Verification items for this drawing (mm, ordinates from the low corner). Round coordinates to 2 decimals unless told otherwise and drop trailing zeros. Loops run counter-clockwise (first coordinate to the right, second up) from the corner with the lowest first, then second, coordinate; pieces in that order, holes last. Notation, with made-up numbers: (69.5, -32) - (103.5, -32) arc R21 ccw to (103.5, -9) - close; hole circle Ø3 at (-33.75, 74). An arc over 180 degrees is marked (long way). Answer in a Markdown table with one row per item. Add a question column.
(1) Mould release check, pull along X, two halves, no side actions. Record for the marked faces 1, 2 and 3: +X half, -X half, draft (parallel to the pull), parting line (faces both ways), or undercut.
(2) Cross-section at D-D on z = 8.5. Enter the section's corners in (x, y), then the cut area to 3 significant figures.
(3) Cross-section at A-A on z = 3. Enter the section's corners in (x, y).
(4) Thickness scan on line 1 along Y through (x, z) = (6, 12); line 2 along Z through (x, y) = (5, 7.25); line 3 along Z through (x, y) = (6.25, 5.75). Record the ranges inside material, lowest first.
(5) Gauge pin test, flat ends, axial feed: pin 1 (2.5 mm diameter, centred on x = 6, y = 6, fed in from +Z); pin 2 (1.5 mm diameter, centred on y = 2.5, z = 8, fed in from +X); pin 3 (3 mm diameter, centred on x = 8, y = 2.5, fed in from -Z). Record the tip position at first contact, or that the pin passes through.
(6) Cross-section at C-C on y = 6. Enter the section's corners in (x, z).
(7) Cross-section at B-B on x = 6. Enter the section's corners in (y, z).
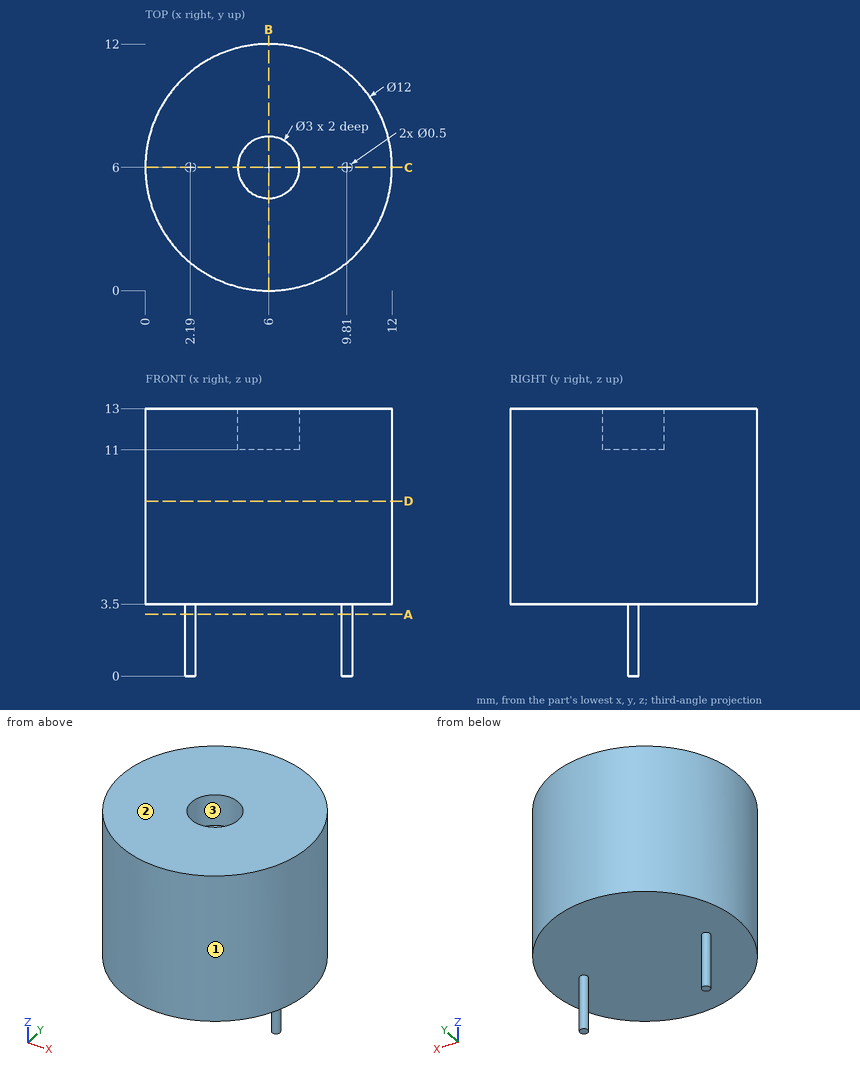
Answers:
| question | item | result |
|---|---|---|
| 1 | face 1 | parting line |
| 1 | face 2 | draft |
| 1 | face 3 | undercut |
| 2 | outline | circle Ø12 at (6, 6) |
| 2 | area | 113 mm^2 |
| 3 | outline | circle Ø0.5 at (2.19, 6); circle Ø0.5 at (9.81, 6) |
| 4 | line 1 | y = 0 to 4.5, 7.5 to 12 |
| 4 | line 2 | z = 3.5 to 13 |
| 4 | line 3 | z = 3.5 to 11 |
| 5 | pin 1 | stops at z = 11 |
| 5 | pin 2 | stops at x = 11.33 |
| 5 | pin 3 | stops at z = 3.5 |
| 6 | outline | (0, 3.5) - (1.94, 3.5) - (1.94, 0) - (2.44, 0) - (2.44, 3.5) - (9.56, 3.5) - (9.56, 0) - (10.06, 0) - (10.06, 3.5) - (12, 3.5) - (12, 13) - (7.5, 13) - (7.5, 11) - (4.5, 11) - (4.5, 13) - (0, 13) - close |
| 7 | outline | (0, 3.5) - (12, 3.5) - (12, 13) - (7.5, 13) - (7.5, 11) - (4.5, 11) - (4.5, 13) - (0, 13) - close |
